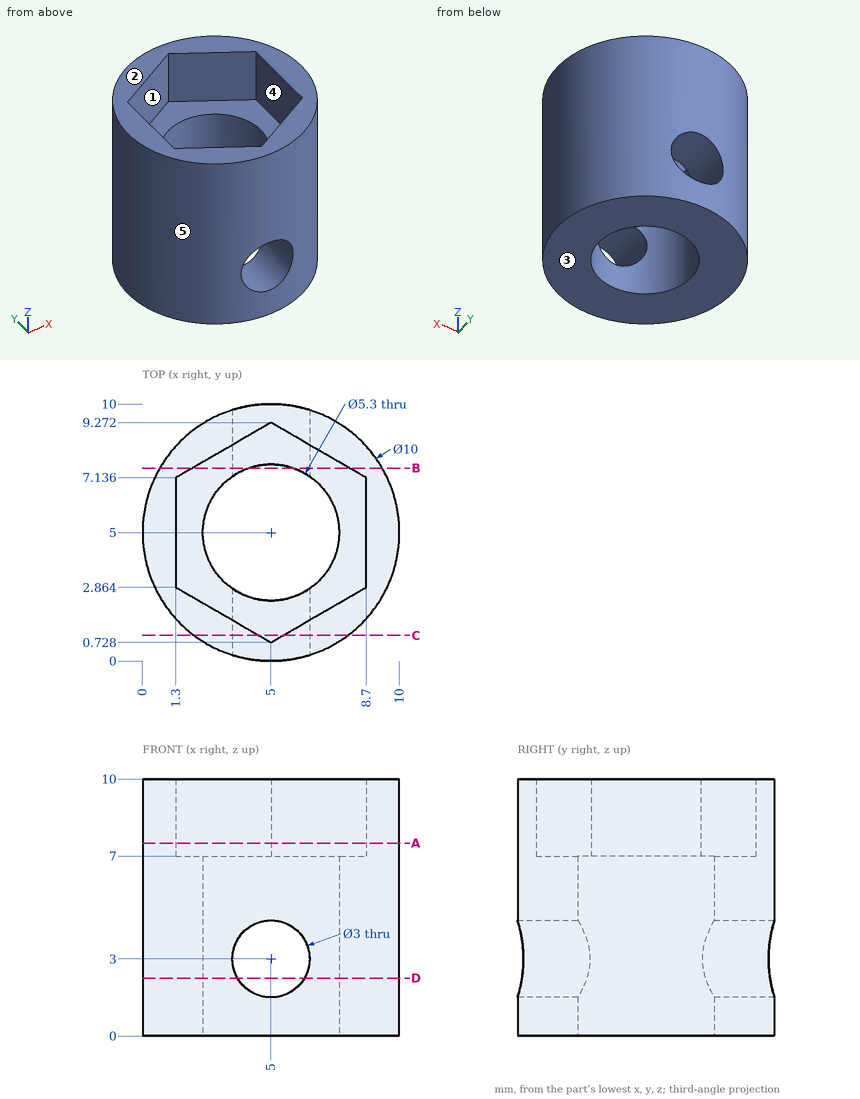
Answer from the drawing. Dimensions are ordinates in mm from the lowest x, y and z of the part. A direction names the side the tool comes from. Give positions to 0.01 mm unless a question says otherwise; leave off trailing zeros. Write each loop counter-clockwise with the first axis right and the second up, starting at its lowest first coordinate (ties: lowest second). Pieces come first, ordered by that corner, then holes. Notation, with made-up numbers: (63.5, 71.25) - (94.5, 71.25) arc R26 ccw to (94.5, 94.25) - close; hole circle Ø5 at (79, 19.25). An arc over 180 degrees is marked (long way). One line per item, written item: value. Start each with the question number.
1. Find section B-B (y = 7.5). Write down the section's boundary in (x, z) (1 decimal).
2. Consider probe 1 along Y at (x, z) = (5, 5.25); probe 2 along Z at (x, y) = (7.75, 4.5); probe 3 along X at (y, z) = (5.25, 8). Determine where each line is inside the solid, lowest interval first.
3. Given pin 1 (0.9 mm diameter, centred on y = 6, z = 9, fed in from -X); pin 2 (6 mm diameter, centred on x = 7, z = 1.5, fed in from -Y); pin 3 (3.5 mm diameter, centred on x = 5, y = 4, fed in from +Z); pin 4 (3 mm diameter, centred on y = 3, z = 2, fed in from +X) (1 decimal), each flat-ended and moving along its own axis, determine where each tip first touches the part or whether it passes through.
4. For the marked faces 1 and 2, determine the directions among +Z, -Z, +X, -X, +Y, -Y from which every point of the face is accessible in a straight line to the end or side of a thin tool.
5. Find section A-A (z = 7.5). Write down the section's boundary in (x, y).
6. For a pull along Y with two mould halves and no side action, classify the marked faces 3, 4 and 5 as +Y half, -Y half, draft (parallel to the pull), parting line (faces both ways), or undercut.
7. Find section D-D (z = 2.25). Write down the section's boundary in (x, y), then the cut area to 3 significant figures.
8. Find section C-C (y = 1). Write down the section's boundary in (x, z).
Geometry results:
1. outline: (0.7, 0) - (4.1, 0) - (4.1, 1.8) arc R1.5 cw to (4.1, 4.2) - (4.1, 7) - (1.9, 7) - (1.9, 10) - (0.7, 10) - close; (5.9, 0) - (9.3, 0) - (9.3, 10) - (8.1, 10) - (8.1, 7) - (5.9, 7) - (5.9, 4.2) arc R1.5 cw to (5.9, 1.8) - close
2. probe 1: 0 to 2.35, 7.65 to 10
2. probe 2: 0 to 7
2. probe 3: 0.01 to 1.3, 8.7 to 9.99
3. pin 1: x = 0.03
3. pin 2: y = 0
3. pin 3: z = 7
3. pin 4: x = 10
4. face 1: +Z
4. face 2: +Z, +X, -X, +Y, -Y
5. outline: circle Ø10 at (5, 5); hole (1.3, 2.86) - (5, 0.73) - (8.7, 2.86) - (8.7, 7.14) - (5, 9.27) - (1.3, 7.14) - close
6. face 3: draft
6. face 4: undercut
6. face 5: parting line
7. outline: (3.7, 0.17) - (3.7, 2.69) arc R2.65 cw to (3.7, 7.31) - (3.7, 9.83) arc R5 ccw to start; (6.3, 0.17) arc R5 ccw to (6.3, 9.83) - (6.3, 7.31) arc R2.65 cw to (6.3, 2.69) - close
7. area: 44.0 mm2
8. outline: (2, 0) - (8, 0) - (8, 10) - (5.47, 10) - (5.47, 7) - (4.53, 7) - (4.53, 10) - (2, 10) - close; hole circle Ø3 at (5, 3)
